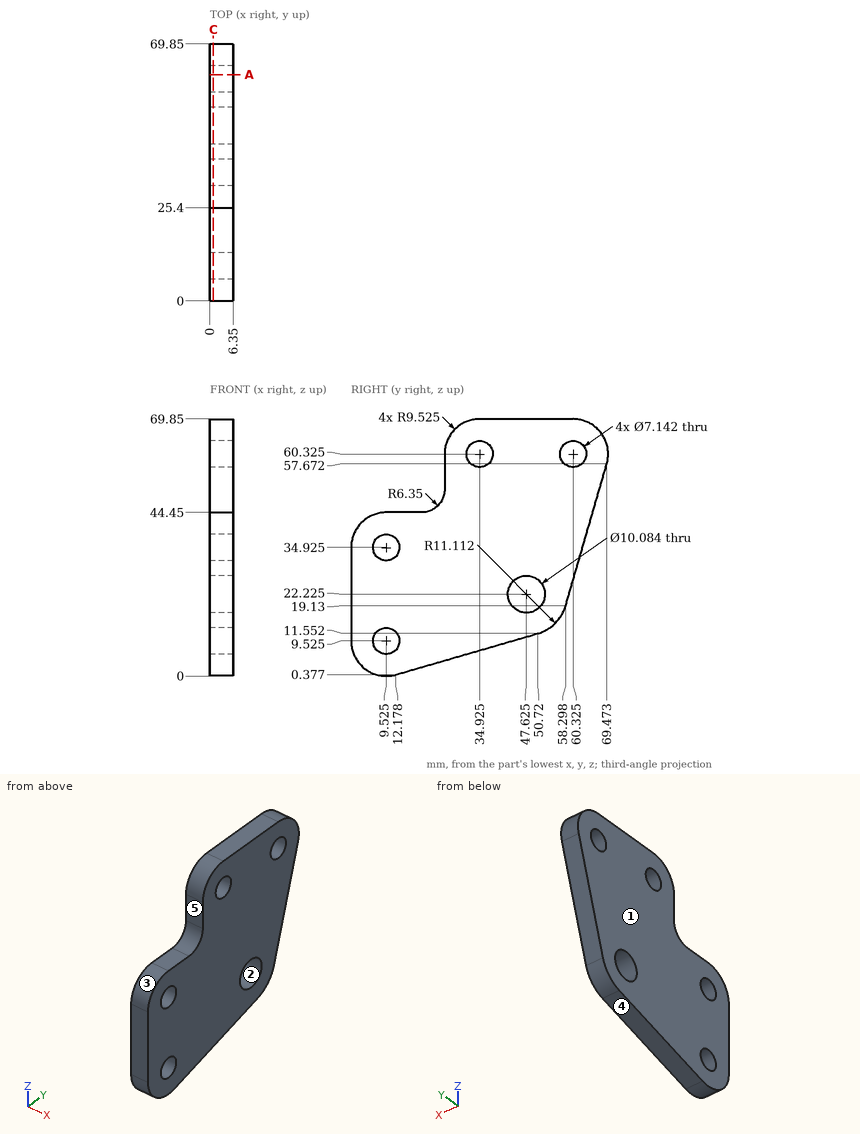
Source: three-view drawing plus pictorial views. Frame: mm from the lowest corner of the part. A direction names the side the tool comes from. Give positions to 0.01 mm unless a question says otherwise; leave off trailing zeros. Write each loop counter-clockwise with the first axis right and the second up, starting at its lowest first coordinate (ties: lowest second). Pieces come first, ordered by that corner, then holes. Notation, with made-up numbers: (27.5, 32) -> (48.5, 32) arc R21 ccw to (48.5, 43) -> close; hole circle Ø11 at (23, -27.5). An arc over 180 degrees is marked (long way). Write item = value, one per line.
Q1. First-contact query: pin 1 (3 mm diameter, centred on x = 5, y = 31, fed in from -Z); pin 2 (4.5 mm diameter, centred on y = 9.525, z = 9.525, fed in from -X). Flat tips, straight axial feed; report the tip coordinate or a pass-through.
Here are the results:
pin_1 = 5.4
pin_2 = through
Q2. Line query: line 1 (Z direction, x = 3, y = 10.5); line 2 (Y direction, x = 5.75, z = 33) (1 decimal); line 3 (Y direction, x = 5.25, z = 36). Output: solid intervals per line, ascending. Write a range as from..to.
Here are the results:
line_1 = 0.05..6.09, 12.96..31.49, 38.36..44.45
line_2 = 0..6.5, 12.5..62.3
line_3 = 0.06..6.12, 12.93..63.19
Q3. Mould query, pull axis Z, two halves, no side actions, for the marked faces 1, 2 and 3. Classes: +Z half, -Z half, draft (parallel to the pull), parting line (faces both ways), or undercut.
Here are the results:
face_1 = draft
face_2 = undercut
face_3 = +Z half
Q4. Reachability of the marked faces 4 and 5 from +Z, -Z, +X, -X, +Y, -Y: full face, straight path, thin tool, end or side. Return the list, or none.
Here are the results:
face_4 = -Z, +X, -X, +Y
face_5 = +Z, +X, -X, -Y
Q5. Cut plane A-A on y = 61.5. Return loops of the section in (x, z).
Here are the results:
outline = (0, 30.17) -> (6.35, 30.17) -> (6.35, 56.95) -> (0, 56.95) -> close; (0, 63.7) -> (6.35, 63.7) -> (6.35, 69.78) -> (0, 69.78) -> close
Q6. Cut plane C-C on x = 1. State how many separate pieces and enclosed holes the cut face has, then the cut area to 3 significant figures.
Here are the results:
separate_pieces = 1
enclosed_holes = 5
area = 3,140 mm²
